Can you work these out from the model? Positions are in its coordinate system, mm. Face numbers are marked on the shaded views. A direction names the side the tool comes from. Coordinates: 2 decimals unless noted, no trailing zeros. Loops run counter-clockwise (first coordinate to the right, second up) from the corner with the lowest first, then second, coordinate; pieces in that order, holes last. Notation, with made-up numbers: M 51.25,-16.75 L 96.25,-16.75 A23 cw 96.25,20.25 Z; hole C 22.5,88 d10. An arc over 180 degrees is marked long. Return JSON: item names as keys, results as strings. Group by question number.
```python
from build123d import *

# Parameters (mm, degrees)
F0_W      = 29
F0_H      = 16.5
F1_DEPTH  = 38.5
F2_T      = -2
F3_DEPTH  = 2.25
F4_SIZE   = 2
F5_SIZE   = 2
F6_SIZE   = 1
F8_DEPTH  = 16.501
F9_W      = 7.54
F9_H      = 7.25
F9_R      = 1.1
F10_DEPTH = 6.35
F13_W     = 5.538
F13_H     = 4.583
F11_W     = 5.538
F11_H     = 5.533


with BuildPart() as f1:
    # F0 (on Top) → F1 (new body)
    with BuildSketch(Plane.XY):
        with Locations((14.5, 8.25)):
            Rectangle(F0_W, F0_H)
    extrude(amount=F1_DEPTH)

    # F2
    f2_openings = [f1.faces().sort_by_distance(p)[0] for p in [
        (14.5, 8.25, 38.5),
    ]]
    offset(amount=F2_T, openings=f2_openings)

    # F3 (add): a face of the model
    f3_faces = [f1.faces().sort_by_distance(p)[0] for p in [
        (14.5, 8.25, 2),
    ]]
    extrude(f3_faces, amount=F3_DEPTH)

    # F4
    f4_edges = [f1.edges().sort_by_distance(p)[0] for p in [
        (29, 0, 19.25),
        (29, 16.5, 19.25),
        (0, 0, 19.25),
        (0, 16.5, 19.25),
    ]]
    chamfer(f4_edges, length=F4_SIZE)

    # F5
    f5_edges = [f1.edges().sort_by_distance(p)[0] for p in [
        (14.5, 0, 0),
        (28, 1, 0),
        (29, 8.25, 0),
        (28, 15.5, 0),
        (14.5, 16.5, 0),
        (1, 15.5, 0),
        (0, 8.25, 0),
        (1, 1, 0),
    ]]
    chamfer(f5_edges, length=F5_SIZE)

    # F6
    f6_edges = [f1.edges().sort_by_distance(p)[0] for p in [
        (0, 8.25, 38.5),
        (1, 1, 38.5),
        (14.5, 0, 38.5),
        (28, 1, 38.5),
        (29, 8.25, 38.5),
        (28, 15.5, 38.5),
        (14.5, 16.5, 38.5),
        (1, 15.5, 38.5),
    ]]
    chamfer(f6_edges, length=F6_SIZE)

    # F7 (on face) → F8 (cut, through all)
    with BuildSketch(Plane(origin=(0, 16.5, 0), x_dir=(-1, 0, 0), z_dir=(0, 1, 0))):
        Polygon((-22.536, 8.664), (-22.536, 4.94), (-5.464, 4.94), (-5.464, 8.664), (-11.635, 12.834), (-16.365, 12.834), align=None)
    extrude(amount=-F8_DEPTH, mode=Mode.SUBTRACT)

    # F9 (on face) → F10 (join)
    with BuildSketch(Plane.YZ.offset(29)):
        with Locations((8.25, 7.875)):
            Rectangle(F9_W, F9_H)
        with Locations((8.25, 9)):
            Circle(F9_R, mode=Mode.SUBTRACT)
    extrude(amount=-F10_DEPTH)

    # F13 (on offset) → F14 section 0
    with BuildSketch(Plane.YZ.offset(24.55)):
        with Locations((8.25, 8.5135)):
            Rectangle(F13_W, F13_H)
    # F11 (on face) → F14 section 1
    with BuildSketch(Plane.YZ.offset(29)):
        with Locations((8.25, 8.0385)):
            Rectangle(F11_W, F11_H)
    loft(mode=Mode.SUBTRACT)


solid = f1.part
```
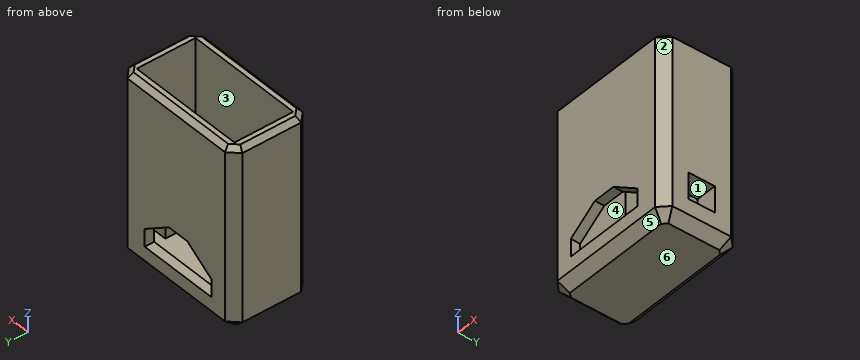
1) Suppose I cut it at B-B, the plane y = 8.25. List the corners of the cut face in (x, z) for me (3 decimals).
2) Suppose I cut it at D-D, the plane y = 5. List the corners of the cut face in (x, z) for me, then the cut area to 3 significant figures.
3) If we mould it in two halves opening along Y, with no side actions, what happens to the marked faces 4, 5 and 6? For each: +Y half, -Y half, draft (parallel to the pull), parting line (faces both ways), or undercut.
4) Suppose I cut it at C-C, the plane z = 17.5. List the corners of the cut face in (x, y) for me, then the cut area to 3 significant figures.
5) For pin 1 (1.3 mm diameter, centred on y = 8.25, z = 9, fed in from +X); pin 2 (2 mm diameter, centred on x = 13.5, y = 0.5, fed in from -Z); pin 3 (0.6 mm diameter, centred on y = 1, z = 7, fed in from -X), each with a flat end and sliding along its axis, tell me the tip position at first contact or that it passes through.
6) For the marked faces 1, 2 and 3, which set-ups out of +Z, -Z, +X, -X, +Y, -Y let a thin tool reach every point of the face, with its end or its side?
7) If I drill on line 1 (X direction, y = 8.25, z = 10.5); line 2 (Y direction, x = 6, z = 15.5); line 3 (X direction, y = 3, z = 10.5), over which ranges is the centre line in solid material (lowest first)? Write a range as from..to.
8) Suppose I cut it at A-A, the plane x = 15.75. List the corners of the cut face in (y, z) for me.
Returned:
{
 "1": {"outline": "M 0,2 L 2,0 L 27,0 L 29,2 L 29,5.272 L 24.55,6.222 L 24.55,7.9 L 22.65,7.9 L 22.65,4.25 L 2,4.25 L 2,38.5 L 1,38.5 L 0,37.5 Z; M 22.65,10.1 L 24.55,10.1 L 24.55,10.805 L 29,10.805 L 29,37.5 L 28,38.5 L 27,38.5 L 27,11.5 L 22.65,11.5 Z"},
 "2": {"outline": "M 0,2 L 2,0 L 27,0 L 29,2 L 29,37.5 L 28,38.5 L 27,38.5 L 27,11.5 L 22.65,11.5 L 22.65,4.25 L 2,4.25 L 2,38.5 L 1,38.5 L 0,37.5 Z", "area": "287 mm²"},
 "3": {"face 4": "undercut", "face 5": "-Y half", "face 6": "draft"},
 "4": {"outline": "M 0,2 L 2,0 L 27,0 L 29,2 L 29,14.5 L 27,16.5 L 2,16.5 L 0,14.5 Z; hole M 2,2 L 27,2 L 27,14.5 L 2,14.5 Z", "area": "158 mm²"},
 "5": {"pin 1": "stops at x = 2", "pin 2": "stops at z = 0.5", "pin 3": "stops at x = 0.7"},
 "6": {"face 1": "+X", "face 2": "+Z, -Z, +X, -Y", "face 3": "+Z"},
 "7": {"line 1": "x = 0..2, 22.65..24.55", "line 2": "y = 0..2, 14.5..16.5", "line 3": "x = 0..2, 27..29"},
 "8": {"outline": "M 0,2 L 2,0 L 14.5,0 L 16.5,2 L 16.5,4.94 L 14.5,4.94 L 14.5,4.25 L 2,4.25 L 2,4.94 L 0,4.94 Z; M 0,12.83 L 2,12.83 L 2,38.5 L 1,38.5 L 0,37.5 Z; M 14.5,12.83 L 16.5,12.83 L 16.5,37.5 L 15.5,38.5 L 14.5,38.5 Z"}
}
